```python
from build123d import *

# Parameters (mm, degrees)
SKETCH_1_W                   = 100
SKETCH_1_H                   = 100
EXTRUDE_1_DEPTH              = 7.75
SKETCH_2_R                   = 30.5
CUT_EXTRUDE_1_DEPTH          = 17
SKETCH_3_W                   = 100
SKETCH_3_H                   = 100
SKETCH_3_R                   = 34
CUT_EXTRUDE_2_DEPTH          = 2
SKETCH_4_W                   = 100
SKETCH_4_H                   = 100
SKETCH_4_R                   = 47.5
CUT_EXTRUDE_3_DEPTH          = 1.5
HOLE_WIZARD_M6_1_D           = 6
HOLE_WIZARD_M6_1_CBORE_D     = 10
HOLE_WIZARD_M6_1_CBORE_DEPTH = 6
PATTERN_CIRCULAR_1_COUNT     = 8
CUT_EXTRUDE_4_REACH          = 74.083
SKETCH_8_R                   = 5.5


with BuildPart() as part:
    # 草图1 → 凸台-拉伸1 (new, symmetric)
    with BuildSketch(Plane.XY):
        Rectangle(SKETCH_1_W, SKETCH_1_H)
    extrude(amount=EXTRUDE_1_DEPTH, both=True)

    # 草图2 → 切除-拉伸1 (cut)
    with BuildSketch(Plane.XY.offset(7.75)):
        Circle(SKETCH_2_R)
    extrude(amount=-CUT_EXTRUDE_1_DEPTH, mode=Mode.SUBTRACT)

    # 草图3 → 切除-拉伸2 (cut)
    with BuildSketch(Plane.XY.offset(7.75)):
        Rectangle(SKETCH_3_W, SKETCH_3_H)
        Circle(SKETCH_3_R, mode=Mode.SUBTRACT)
    extrude(amount=-CUT_EXTRUDE_2_DEPTH, mode=Mode.SUBTRACT)

    # 草图4 → 切除-拉伸3 (cut)
    with BuildSketch(Plane(origin=(0, 0, -7.75), x_dir=(-1, 0, 0), z_dir=(0, 0, -1))):
        Rectangle(SKETCH_4_W, SKETCH_4_H)
        Circle(SKETCH_4_R, mode=Mode.SUBTRACT)
    extrude(amount=-CUT_EXTRUDE_3_DEPTH, mode=Mode.SUBTRACT)

    # M6 六角头螺栓的柱形沉头孔1 (through all)
    with Locations(Plane(origin=(0, 0, -7.75), x_dir=(-1, 0, 0), z_dir=(0, 0, -1))):
        with Locations((0, 38)):
            hole_wizard_m6_1 = CounterBoreHole(HOLE_WIZARD_M6_1_D / 2, HOLE_WIZARD_M6_1_CBORE_D / 2, HOLE_WIZARD_M6_1_CBORE_DEPTH)

    # 阵列(圆周)1: M6 六角头螺栓的柱形沉头孔1 ×8 about axis
    pattern_circular_1_axis = Axis((0, 0, 0), (0, 0, 1))
    for i in range(1, PATTERN_CIRCULAR_1_COUNT):
        add(hole_wizard_m6_1.rotate(pattern_circular_1_axis, i * 360 / PATTERN_CIRCULAR_1_COUNT), mode=Mode.SUBTRACT)

    # 草图8 → 切除-拉伸4 (cut, up to next)
    with BuildSketch(Plane(origin=(0, 0, -6.25), x_dir=(-1, 0, 0), z_dir=(0, 0, -1)), mode=Mode.PRIVATE) as cut_extrude_4_sk1:
        with Locations((40, 40)):
            Circle(SKETCH_8_R)
    cut_extrude_4_tool1 = extrude(cut_extrude_4_sk1.sketch, amount=-CUT_EXTRUDE_4_REACH, mode=Mode.PRIVATE) & part.part
    # 草图8 → 切除-拉伸4 (cut, up to next)
    with BuildSketch(Plane(origin=(0, 0, -6.25), x_dir=(-1, 0, 0), z_dir=(0, 0, -1)), mode=Mode.PRIVATE) as cut_extrude_4_sk2:
        with Locations((40, -40)):
            Circle(SKETCH_8_R)
    cut_extrude_4_tool2 = extrude(cut_extrude_4_sk2.sketch, amount=-CUT_EXTRUDE_4_REACH, mode=Mode.PRIVATE) & part.part
    # 草图8 → 切除-拉伸4 (cut, up to next)
    with BuildSketch(Plane(origin=(0, 0, -6.25), x_dir=(-1, 0, 0), z_dir=(0, 0, -1)), mode=Mode.PRIVATE) as cut_extrude_4_sk3:
        with Locations((-40, -40)):
            Circle(SKETCH_8_R)
    cut_extrude_4_tool3 = extrude(cut_extrude_4_sk3.sketch, amount=-CUT_EXTRUDE_4_REACH, mode=Mode.PRIVATE) & part.part
    # 草图8 → 切除-拉伸4 (cut, up to next)
    with BuildSketch(Plane(origin=(0, 0, -6.25), x_dir=(-1, 0, 0), z_dir=(0, 0, -1)), mode=Mode.PRIVATE) as cut_extrude_4_sk4:
        with Locations((-40, 40)):
            Circle(SKETCH_8_R)
    cut_extrude_4_tool4 = extrude(cut_extrude_4_sk4.sketch, amount=-CUT_EXTRUDE_4_REACH, mode=Mode.PRIVATE) & part.part
    add(cut_extrude_4_tool1.solids().sort_by_distance((-40, 40, -6.25))[0], mode=Mode.SUBTRACT)
    add(cut_extrude_4_tool2.solids().sort_by_distance((-40, -40, -6.25))[0], mode=Mode.SUBTRACT)
    add(cut_extrude_4_tool3.solids().sort_by_distance((40, -40, -6.25))[0], mode=Mode.SUBTRACT)
    add(cut_extrude_4_tool4.solids().sort_by_distance((40, 40, -6.25))[0], mode=Mode.SUBTRACT)


solid = part.part
```
Here's how the part is built. I have some questions about the finished solid (model axes, mm). A direction names the side the tool comes from. Coordinates: 2 decimals unless noted, no trailing zeros. Loops run counter-clockwise (first coordinate to the right, second up) from the corner with the lowest first, then second, coordinate; pieces in that order, holes last. Notation, with made-up numbers: (1, -2) - (14, -2) arc R16 cw to (14, 29) - close; hole circle Ø4 at (-7, 77). An arc over 180 degrees is marked (long way). Answer as CSV lines item,"result".
Q1. We'd pull the mould along Y, two halves only. Please class faces 3 (the face through (-1, 50, 0)), 4 (the face through (10.3, -46.37, -7.01)), 5 (the face through (0, -41, 2)): pulls with the +Y half, pulls with the -Y half, needs draft (parallel to the pull), parting line crosses it, or undercut.
Response:
face 3,"pulls with the +Y half"
face 4,"parting line crosses it"
face 5,"undercut"
Q2. If we section it at C-C, the plane z = -4.75: Give the number of separate pieces and of enclosed holes in the cut face, and give its area (3 significant figures).
Response:
separate pieces,"1"
enclosed holes,"13"
area,"6,070 mm2"
Q3. For pin 1 (3.5 mm diameter, centred on x = 26.87, y = 26.87, fed in from -Z); pin 2 (3 mm diameter, centred on x = -26, y = -29, fed in from -Z), each with a flat end and sliding along its axis, tell me the tip position at first contact or that it passes through.
Response:
pin 1,"through"
pin 2,"z = -1.75"
Q4. If I drill on L1, parallel to Y at x = 40, z = 0; L2, parallel to X at y = -27.5, z = -3.75; L3, parallel to Z at x = -16.5, y = -38.5, over which ranges is the centre line in solid material (lowest first)? Write a range as [from, to].
Response:
L1,"[-50, -45.5], [-34.5, -2.24], [2.24, 34.5], [45.5, 50]"
L2,"[-50, -31.83], [-21.91, -13.19], [13.19, 21.91], [31.83, 50]"
L3,"[-7.75, 5.75]"
Q5. If we section it at A-A, the plane x = 36.5: Write out the boundary of the cut face in (y, z).
Response:
outline,"(-50, -6.25) - (-44.24, -6.25) - (-44.24, 5.75) - (-50, 5.75) - close; (-35.76, -6.25) - (-30.4, -6.25) - (-30.4, -7.75) - (-4.77, -7.75) - (-4.77, -1.75) - (-2.6, -1.75) - (-2.6, 5.75) - (-35.76, 5.75) - close; (2.6, -1.75) - (4.77, -1.75) - (4.77, -7.75) - (30.4, -7.75) - (30.4, -6.25) - (35.76, -6.25) - (35.76, 5.75) - (2.6, 5.75) - close; (44.24, -6.25) - (50, -6.25) - (50, 5.75) - (44.24, 5.75) - close"
Q6. For faces 1 (the face through (24.84, 29.08, 2.05)), 2 (the face through (-24.6, -29.2, -1.75)), which set-ups out of +Z, -Z, +X, -X, +Y, -Y let a thin tool reach every point of the face, with its end or its side?
Response:
face 1,"+Z, -Z"
face 2,"-Z"
Q7. If we section it at D-D, the plane y = -7: Write out the boundary of the cut face in (x, z), and give its area (3 significant figures).
Response:
outline,"(-50, -6.25) - (-46.98, -6.25) - (-46.98, -7.75) - (-29.69, -7.75) - (-29.69, 7.75) - (-33.27, 7.75) - (-33.27, 5.75) - (-50, 5.75) - close; (29.69, -7.75) - (46.98, -7.75) - (46.98, -6.25) - (50, -6.25) - (50, 5.75) - (33.27, 5.75) - (33.27, 7.75) - (29.69, 7.75) - close"
area,"554 mm2"
